Geometry check sheet. Reference: the model listing, model coordinates, mm. A direction names the side the tool comes from. Coordinates: 2 decimals unless noted, no trailing zeros. Loops run counter-clockwise (first coordinate to the right, second up) from the corner with the lowest first, then second, coordinate; pieces in that order, holes last.
from build123d import *

# Parameters (mm, degrees)
F0_W      = 115
F0_H      = 170
F1_DEPTH  = 12
F2_W      = 95
F2_H      = 150
F3_DEPTH  = 12.001
F4_R      = 1.55
F5_DEPTH  = 12.001
F6_R      = 4
F7_R      = 1.55
F8_DEPTH  = 12.001
F9_R      = 4
F10_DEPTH = 5


with BuildPart() as f1:
    # F0 (on Top) → F1 (new body)
    with BuildSketch(Plane.XY):
        Rectangle(F0_W, F0_H)
    extrude(amount=F1_DEPTH)

    # F2 (on face) → F3 (cut, through all)
    with BuildSketch(Plane.XY.offset(12)):
        Rectangle(F2_W, F2_H)
    extrude(amount=-F3_DEPTH, mode=Mode.SUBTRACT)

    # F4 (on face) → F5 (cut, through all)
    with BuildSketch(Plane.XY.offset(12)):
        with Locations((0, 80)):
            Circle(F4_R)
        with Locations((0, -80)):
            Circle(F4_R)
        with Locations((52.5, 0)):
            Circle(F4_R)
        with Locations((-52.5, 0)):
            Circle(F4_R)
    extrude(amount=-F5_DEPTH, mode=Mode.SUBTRACT)

    # F6
    f6_edges = [f1.edges().sort_by_distance(p)[0] for p in [
        (47.5, 75, 6),
        (-47.5, 75, 6),
        (57.5, 85, 6),
        (57.5, -85, 6),
        (-57.5, -85, 6),
        (-57.5, 85, 6),
        (47.5, -75, 6),
        (-47.5, -75, 6),
    ]]
    fillet(f6_edges, radius=F6_R)

    # F7 (on face) → F8 (cut, through all)
    with BuildSketch(Plane.XY.offset(12)):
        with Locations((-49.75, 77.25)):
            Circle(F7_R)
        with Locations((49.75, 77.25)):
            Circle(F7_R)
        with Locations((49.75, -77.25)):
            Circle(F7_R)
        with Locations((-49.75, -77.25)):
            Circle(F7_R)
    extrude(amount=-F8_DEPTH, mode=Mode.SUBTRACT)

    # F9 (on face) → F10 (cut)
    with BuildSketch(Plane.XY.offset(12)):
        with Locations((0, 80)):
            Circle(F9_R)
        with Locations((-52.5, 0)):
            Circle(F9_R)
        with Locations((0, -80)):
            Circle(F9_R)
        with Locations((52.5, 0)):
            Circle(F9_R)
    extrude(amount=-F10_DEPTH, mode=Mode.SUBTRACT)


solid = f1.part
(1) Scan lines: L1, parallel to X at y = 77.25, z = 6.5; L2, parallel to Y at x = 0, z = 8.45; L3, parallel to X at y = -13, z = 11.25. Record each from-to range of solid material in increasing order.
Findings:
L1: x = -57.5 to -51.3, -48.2 to 48.2, 51.3 to 57.5
L2: y = -85 to -84, -76 to -75, 75 to 76, 84 to 85
L3: x = -57.5 to -47.5, 47.5 to 57.5
(2) Sectioned sample at B-B on z = 2. State how many separate pieces and enclosed holes the cut face has, and give its area (3 significant figures).
Findings:
separate pieces: 1
enclosed holes: 9
area: 5,240 mm2
(3) Draft check along X on faces 4 (the cylindrical face through (56.297, 83.859, 6.084)), 5 (the flat face through (0, 78, 7)), 6 (the flat face through (50.8, 0.4, 0)), 7 (the flat face through (-57.5, -1, 6)). Enter one of: +X half, -X half, draft (parallel to the pull), parting line (faces both ways), or undercut.
Findings:
face 4: +X half
face 5: undercut
face 6: draft
face 7: -X half
(4) Gauge pin test, flat ends, axial feed: pin 1 Ø3 at (x, y) = (49.75, 77.25) entering from +Z; pin 2 Ø4 at (x, y) = (-53.5, 1.5) entering from +Z. Record the tip position at first contact, or that the pin passes through.
Findings:
pin 1: passes through
pin 2: stops at z = 7
(5) Access from +Z, -Z, +X, -X, +Y, -Y to the whole of each face (thin tool, end or side, straight path). Record for faces 1 (the flat face through (57.5, -1, 6)), 2 (the flat face through (-1, 75, 6)), 3 (the cylindrical face through (-0.867, -83.905, 9.535)).
Findings:
face 1: +Z, -Z, +X, +Y, -Y
face 2: +Z, -Z
face 3: +Z
(6) Sectioned sample at C-C on y = 62. Record the cut outline in (x, z).
Findings:
outline: (-57.5, 0) - (-47.5, 0) - (-47.5, 12) - (-57.5, 12) - close; (47.5, 0) - (57.5, 0) - (57.5, 12) - (47.5, 12) - close
(7) Sectioned sample at A-A on x = -23. Record the cut outline in (y, z).
Findings:
outline: (-85, 0) - (-75, 0) - (-75, 12) - (-85, 12) - close; (75, 0) - (85, 0) - (85, 12) - (75, 12) - close
